Can you work these out from the drawing? Everything is in mm from the part's minimum corner. A direction names the side the tool comes from. Give positions to 0.01 mm unless a question says otherwise; leave off trailing zeros. Order: outer loops, then holes, each group sorted by start corner. A loop starts at its lowest first (then second) coordinate and runs counter-clockwise, first axis right, second up. Notation, with made-up numbers: M 29.5,88.25 L 86.5,88.25 A8 cw 86.5,95.25 Z; hole C 42,89 d4. An arc over 180 degrees is marked long. Use a Markdown table: item, result. Add a question column.
Item 1: Suppose I cut it at A-A on z = 20.25. Write out the boundary of the cut face in (x, y) (1 decimal), plus the area to 3 significant figures.
Item 2: If I drill on L1, parallel to Z at x = 0.75, y = 1.6; L2, parallel to Y at x = 2.2, z = 17.5; L3, parallel to X at y = 2.85, z = 4.75, over which ranges is the centre line in solid material (lowest first)? Write a range as from..to.
Item 3: If we mould it in two halves opening along Y, with no side actions, what happens to the marked faces 3, 4 and 5? For each: released by +Y, released by -Y, zero draft, split by the parting line, or undercut.
Item 4: Suppose I cut it at B-B on z = 8.5. Write out the boundary of the cut face in (x, y) (1 decimal).
Item 5: I'm going to push flat-ended pins straight in: pin 1 Ø2 at (x, z) = (1.5, 14.5) entering from -Y (1 decimal); pin 2 Ø1.7 at (x, y) = (3.5, 2.5) entering from +Z; pin 3 Ø2 at (x, z) = (3.5, 16) entering from +Y (3 decimals). Where does each tip first touch, or does it pass through?
Item 6: For the marked faces 1 and 2, which set-ups out of +Z, -Z, +X, -X, +Y, -Y let a thin tool reach every point of the face, with its end or its side?
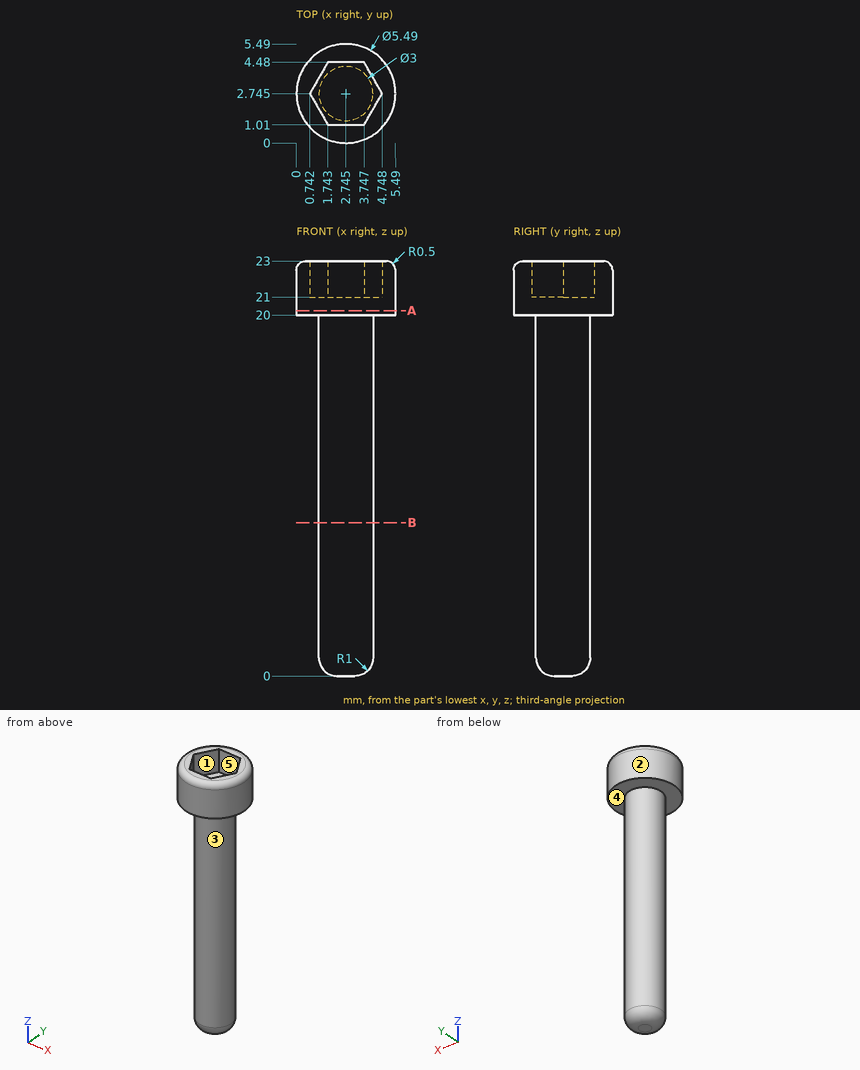
Findings below:
| question | item | result |
|---|---|---|
| 1 | outline | C 2.7,2.7 d5.5 |
| 1 | area | 23.7 mm^2 |
| 2 | L1 | z = 20..23 |
| 2 | L2 | y = 1.35..4.14 |
| 2 | L3 | x = 1.25..4.24 |
| 3 | face 3 | split by the parting line |
| 3 | face 4 | zero draft |
| 3 | face 5 | undercut |
| 4 | outline | C 2.7,2.7 d3 |
| 5 | pin 1 | stops at y = 1.3 |
| 5 | pin 2 | stops at z = 21 |
| 5 | pin 3 | stops at y = 4.245 |
| 6 | face 1 | +Z |
| 6 | face 2 | +Z, -Z |
